Input: dimensioned drawing with shaded views. Units: mm. Origin: part minimum x, y, z. A direction names the side the tool comes from. Give positions to 0.01 mm unless a question says otherwise; leave off trailing zeros. Write each loop counter-clockwise with the first axis right and the second up, starting at its lowest first coordinate (ties: lowest second). Pieces come first, ordered by that corner, then holes. Notation, with made-up numbers: (-33.5, 79.25) - (-23.5, 79.25) arc R17 ccw to (-23.5, 83.25) - close; hole circle Ø4 at (-5, 4). An arc over 180 degrees is marked (long way). Answer as a JSON object with one key per item and string values. Group by question number.
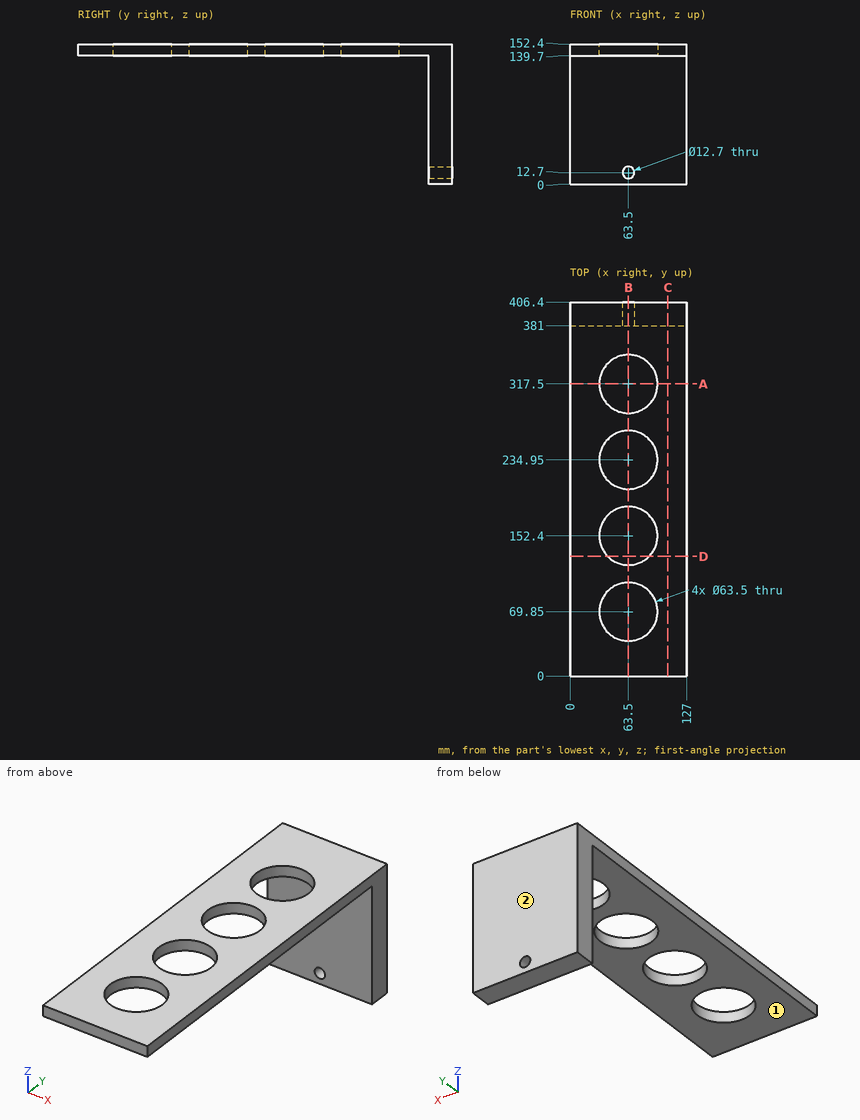
Q1. Reachability of the marked faces 1 and 2 from +Z, -Z, +X, -X, +Y, -Y: full face, straight path, thin tool, end or side. Return the list, or none.
Q2. Ray query, probe 1 along Y at (x, z) = (63, 147); probe 2 along X at (y, z) = (152, 144); probe 3 along Y at (x, z) = (57, 91). Return the intervals inside material, ascending. Write a range as [from, to].
Q3. First-contact query: pin 1 Ø10 at (x, z) = (37, 60.5) entering from -Y; pin 2 Ø7.5 at (x, z) = (63.5, 12.7) entering from -Y. Flat tips, straight axial feed; report the tip coordinate or a pass-through.
Q4. Section B-B on x = 63.5. Return the cut outline in (y, z).
Q5. Section D-D on y = 130. Return the cut outline in (x, z).
Q6. Section A-A on y = 317.5. Return the cut outline in (x, z).
Q7. Section C-C on x = 106.5. Return the cut outline in (y, z), then the cut area to 3 significant figures.
Taken from the geometry:
{
 "1": {"face 1": "-Z, +X, -X, -Y", "face 2": "+Z, -Z, +X, -X, +Y"},
 "2": {"probe 1": "y = [0, 38.1], [101.6, 120.65], [184.15, 203.2], [266.7, 285.75], [349.25, 406.4]", "probe 2": "x = [0, 31.75], [95.25, 127]", "probe 3": "y = [381, 406.4]"},
 "3": {"pin 1": "stops at y = 381", "pin 2": "passes through"},
 "4": {"outline": "(0, 139.7) - (38.1, 139.7) - (38.1, 152.4) - (0, 152.4) - close; (101.6, 139.7) - (120.65, 139.7) - (120.65, 152.4) - (101.6, 152.4) - close; (184.15, 139.7) - (203.2, 139.7) - (203.2, 152.4) - (184.15, 152.4) - close; (266.7, 139.7) - (285.75, 139.7) - (285.75, 152.4) - (266.7, 152.4) - close; (349.25, 139.7) - (381, 139.7) - (381, 19.05) - (406.4, 19.05) - (406.4, 152.4) - (349.25, 152.4) - close; (381, 0) - (406.4, 0) - (406.4, 6.35) - (381, 6.35) - close"},
 "5": {"outline": "(0, 139.7) - (41, 139.7) - (41, 152.4) - (0, 152.4) - close; (86, 139.7) - (127, 139.7) - (127, 152.4) - (86, 152.4) - close"},
 "6": {"outline": "(0, 139.7) - (31.75, 139.7) - (31.75, 152.4) - (0, 152.4) - close; (95.25, 139.7) - (127, 139.7) - (127, 152.4) - (95.25, 152.4) - close"},
 "7": {"outline": "(0, 139.7) - (381, 139.7) - (381, 0) - (406.4, 0) - (406.4, 152.4) - (0, 152.4) - close", "area": "8,710 mm²"}
}
